```python
from build123d import *

# Parameters (mm, degrees)
EXTRUDE_1_DEPTH          = 2.4
SKETCH_2_OUTSIDE_W       = 15.35
SKETCH_2_OUTSIDE_H       = 16.31
SKETCH_2_OUTSIDE_R       = 3.1
CUT_EXTRUDE_2_DEPTH      = 1.5
CUT_EXTRUDE_2_DRAFT      = -60
MIRROR_1_COPY_1_SKETCH_W = 15.35
MIRROR_1_COPY_1_SKETCH_H = 16.31
MIRROR_1_COPY_1_SKETCH_R = 3.1
MIRROR_1_COPY_1_DEPTH    = 1.5
MIRROR_1_COPY_1_DRAFT    = -60
SKETCH_3_R               = 1.75
CUT_EXTRUDE_3_DEPTH      = 6.30879773


with BuildPart() as part:
    # 草圖1 → 伸長1 (new body)
    with BuildSketch(Plane.XY):
        Polygon((0, 3.579571669), (-3.1, 1.789785834), (-3.1, -1.789785834), (0, -3.579571669), (3.1, -1.789785834), (3.1, 1.789785834), align=None)
    extrude(amount=EXTRUDE_1_DEPTH)


with BuildPart() as cut_extrude_2_tool:
    # 草圖2 outside → 伸長2 (with draft: the straight prism first)
    with BuildSketch(Plane.XY.offset(2.4)):
        Rectangle(SKETCH_2_OUTSIDE_W, SKETCH_2_OUTSIDE_H)
        Circle(SKETCH_2_OUTSIDE_R, mode=Mode.SUBTRACT)
    extrude(amount=-CUT_EXTRUDE_2_DEPTH)
    # 伸長2: the draft: its side faces are tilted about the plane it starts from
    cut_extrude_2_sides = [cut_extrude_2_tool.faces().sort_by_distance(p)[0] for p in [
        (0, -8.155, 1.65),
        (7.675, 0, 1.65),
        (0, 8.155, 1.65),
        (-7.675, 0, 1.65),
        (-3.1, 0, 1.65),
    ]]
    draft(cut_extrude_2_sides, Plane.XY.offset(2.4), CUT_EXTRUDE_2_DRAFT)


with BuildPart() as part_1:
    add(part.part)

    # 伸長2: cut by cut_extrude_2_tool
    add(cut_extrude_2_tool.part, mode=Mode.SUBTRACT)


with BuildPart() as mirror_1_copy_1_tool:
    # 鏡射1 copy 1 sketch → 鏡射1 copy 1 (with draft: the straight prism first)
    with BuildSketch(Plane(origin=(0, 0, 0), x_dir=(1, 0, 0), z_dir=(0, 0, -1))):
        Rectangle(MIRROR_1_COPY_1_SKETCH_W, MIRROR_1_COPY_1_SKETCH_H)
        Circle(MIRROR_1_COPY_1_SKETCH_R, mode=Mode.SUBTRACT)
    extrude(amount=-MIRROR_1_COPY_1_DEPTH)
    # 鏡射1 copy 1: the draft: its side faces are tilted about the plane it starts from
    mirror_1_copy_1_sides = [mirror_1_copy_1_tool.faces().sort_by_distance(p)[0] for p in [
        (0, -8.155, 0.75),
        (7.675, 0, 0.75),
        (0, 8.155, 0.75),
        (-7.675, 0, 0.75),
        (-3.1, 0, 0.75),
    ]]
    draft(mirror_1_copy_1_sides, Plane(origin=(0, 0, 0), x_dir=(1, 0, 0), z_dir=(0, 0, -1)), MIRROR_1_COPY_1_DRAFT)


with BuildPart() as part_2:
    add(part_1.part)

    # 鏡射1 copy 1: cut by mirror_1_copy_1_tool
    add(mirror_1_copy_1_tool.part, mode=Mode.SUBTRACT)

    # 草圖3 → 伸長3 (cut, through all)
    with BuildSketch(Plane.XY.offset(2.4)):
        Circle(SKETCH_3_R)
    extrude(amount=-CUT_EXTRUDE_3_DEPTH, mode=Mode.SUBTRACT)


solid = part_2.part
```
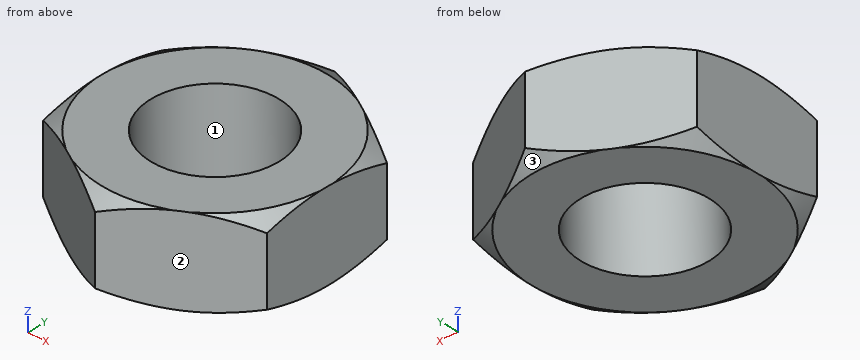
Read the model definition and answer for the solid it produces. Units are mm, in the model's axes. Face numbers are marked on the shaded views. Round coordinates to 2 decimals unless told otherwise and drop trailing zeros. Write each loop counter-clockwise with the first axis right and the second up, starting at its lowest first coordinate (ties: lowest second). Pieces come first, ordered by that corner, then holes. Notation, with made-up numbers: (-10.5, -9.5) - (10.5, -9.5) arc R29 cw to (10.5, 29.5) - close; hole circle Ø2 at (66, 74.5). An arc over 180 degrees is marked (long way). Use CSV: the item, a comma, the result in double quotes.
Q1. Find section A-A, the plane z = 1.8. Write down the section's boundary in (x, y).
Values:
outline,"(-3.1, -1.79) - (0, -3.58) - (3.1, -1.79) - (3.1, 1.79) - (0, 3.58) - (-3.1, 1.79) - close; hole circle Ø3.5 at (0, 0)"
Q2. Determine the mould class of the marked faces 1, 2 and 3 for opening direction Y: +Y half, -Y half, draft (parallel to the pull), parting line (faces both ways), or undercut.
Values:
face 1,"undercut"
face 2,"-Y half"
face 3,"+Y half"
Q3. Straight lines are drawn through the part: line 1 along X through (y, z) = (1, 0.8); line 2 along X through (y, z) = (0.5, 0.85); line 3 along Y through (x, z) = (-0.25, 2). For each, find the intervals that lie inside material, in ascending order.
Values:
line 1,"x = -3.1 to -1.44, 1.44 to 3.1"
line 2,"x = -3.1 to -1.68, 1.68 to 3.1"
line 3,"y = -3.44 to -1.73, 1.73 to 3.44"
Q4. This flat-tipped pin is pushed along its axis until it touches: pin 1 Ø1 at (x, z) = (-2.5, 1.5) entering from -Y. Where does it stop, or does it pass through?
Values:
pin 1,"stops at y = -2.42"
